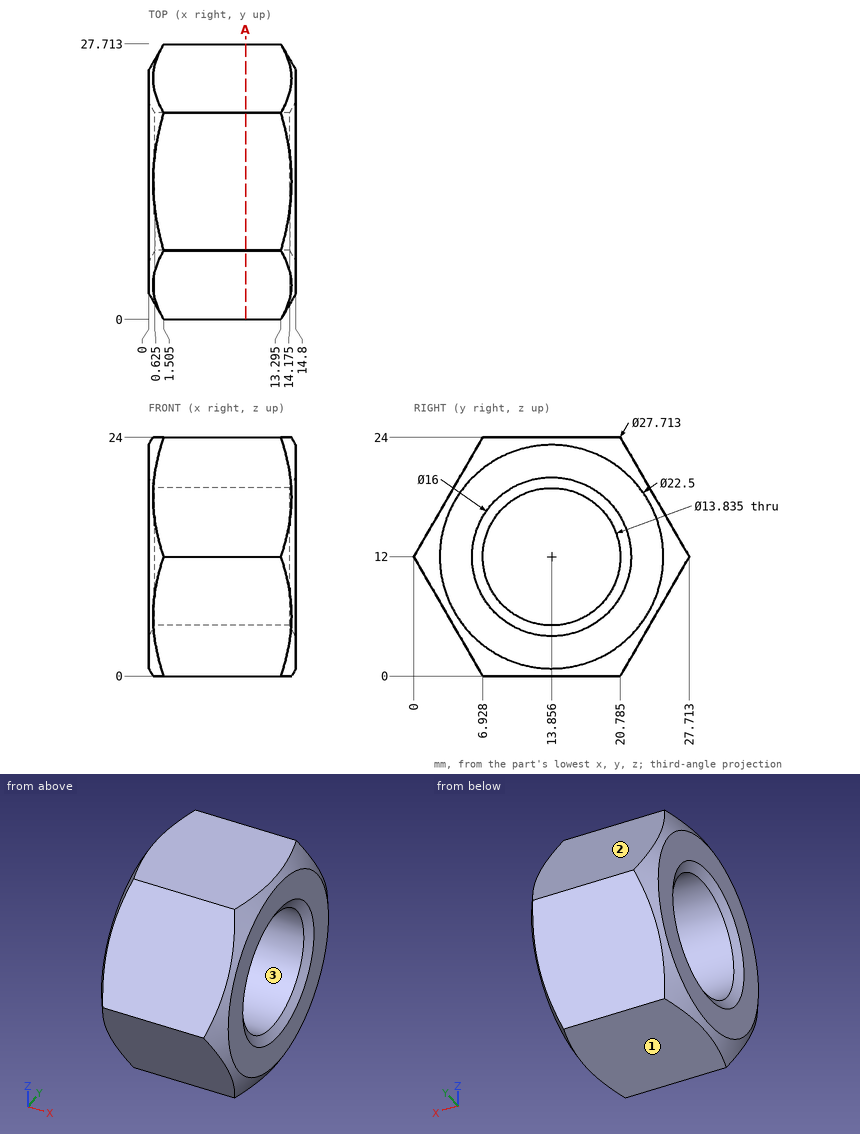
Geometry check sheet. Reference: drawing and pictorial views, mm from the part's lowest x, y, z. Round coordinates to 2 decimals unless told otherwise and drop trailing zeros. Write each loop counter-clockwise with the first axis right and the second up, starting at its lowest first coordinate (ties: lowest second). Pieces come first, ordered by that corner, then holes.
Item 1: Material ranges on line 1 along Z through (x, y) = (4, 17.5); line 2 along Y through (x, z) = (11.75, 16.75) (1 decimal); line 3 along Z through (x, y) = (11.5, 19) (1 decimal), recorded low to high.
Determined:
line 1: z = 0 to 6.12, 17.88 to 24
line 2: y = 2.7 to 8.8, 18.9 to 25
line 3: z = 0 to 7.4, 16.6 to 24
Item 2: Go/stop test with flat-tipped pins: pin 1 Ø1 at (x, z) = (12.5, 6.5) entering from -Y; pin 2 Ø5 at (x, z) = (9.5, 3) entering from -Y; pin 3 Ø5 at (x, y) = (12, 4) entering from -Z. Record where each tip stops, or that it passes through.
Determined:
pin 1: stops at y = 2.89
pin 2: stops at y = 3.75
pin 3: stops at z = 0.74
Item 3: Section check A-A (x = 9.75). Record the boundary of the cut face in (y, z) (1 decimal).
Determined:
outline: (0, 12) - (6.9, 0) - (20.8, 0) - (27.7, 12) - (20.8, 24) - (6.9, 24) - close; hole circle Ø13.8 at (13.9, 12)
Item 4: Mould release check, pull along Z, two halves, no side actions. Record for the marked faces 1, 2 and 3: +Z half, -Z half, draft (parallel to the pull), parting line (faces both ways), or undercut.
Determined:
face 1: -Z half
face 2: +Z half
face 3: undercut
